Source: CAD feature listing. Evaluate the final solid. Frame: model axes, mm. Face numbers are marked on the shaded views. A direction names the side the tool comes from. Coordinates: 2 decimals unless noted, no trailing zeros. Write each loop counter-clockwise with the first axis right and the second up, starting at its lowest first coordinate (ties: lowest second). Pieces come first, ordered by that corner, then holes. Notation, with made-up numbers: (62, 61.25) -> (107, 61.25) arc R31 cw to (107, 99.25) -> close; hole circle Ø5 at (-37, 44.25). An arc over 180 degrees is marked (long way). Write item = value, one per line.
from build123d import *

# Parameters (mm, degrees)
SKIZZE1_W                       = 22.1
SKIZZE1_H                       = 4.3
SCHNITT_LINEAR_START            = -15.1
SKIZZE2_R                       = 7.5
SKIZZE2_R_2                     = 5
SCHNITT_LINEAR_AUSTRAGEN2_DEPTH = 15.1
SCHNITT_LINEAR_START_2          = -3
SCHNITT_LINEAR_AUSTRAGEN4_DEPTH = 3
AUFSATZ_LINEAR_AUSTRAGEN1_DEPTH = 1.5
DURCHGANGSLOCH_F_R_M41_D        = 4.5
VERRUNDUNG3_R                   = 2


with BuildPart() as part:
    # Skizze1 → Rotation1 (revolve)
    with BuildSketch(Plane.XY, mode=Mode.PRIVATE) as rotation1_sk:
        with Locations((11.05, 5.35)):
            Rectangle(SKIZZE1_W, SKIZZE1_H)
    revolve(rotation1_sk.sketch.rotate(Axis((0, 0, 0), (1, 0, 0)), 90), axis=Axis((0, 0, 0), (1, 0, 0)))

    # Skizze2 → Schnitt-Linear austragen2 (cut)
    with BuildSketch(Plane.ZY.offset(SCHNITT_LINEAR_START)):
        Circle(SKIZZE2_R)
        Circle(SKIZZE2_R_2, mode=Mode.SUBTRACT)
    extrude(amount=SCHNITT_LINEAR_AUSTRAGEN2_DEPTH, mode=Mode.SUBTRACT)

    # Skizze3 → Schnitt-Linear austragen4 (cut)
    with BuildSketch(Plane.ZY.offset(-15.1).offset(SCHNITT_LINEAR_START_2)):
        with BuildLine():
            Line((0, 5), (0, 7.5))
            ThreePointArc((0, 7.5), (7.451278665, -0.853490626), (-1.695892399, -7.305747667))
            Line((-1.695892399, -7.305747667), (0.652630961, -4.957224307))
            ThreePointArc((0.652630961, -4.957224307), (4.989294616, 0.327015646), (0, 5))
        make_face()
    extrude(amount=SCHNITT_LINEAR_AUSTRAGEN4_DEPTH, mode=Mode.SUBTRACT)

    # Skizze4 → Aufsatz-Linear austragen1 (add)
    with BuildSketch(Plane(origin=(22.1, 0, 0), x_dir=(0, 0, -1), z_dir=(1, 0, 0))):
        with BuildLine():
            Line((3.348469228, 6.711017347), (3.348469228, 15.5))
            Line((3.348469228, 15.5), (11.348469228, 15.5))
            Line((11.348469228, 15.5), (11.348469228, 9.5))
            Line((11.348469228, 9.5), (7.348469228, 1.5))
            ThreePointArc((7.348469228, 1.5), (5.949352783, 4.566749552), (3.348469228, 6.711017347))
        make_face()
    extrude(amount=-AUFSATZ_LINEAR_AUSTRAGEN1_DEPTH)

    # Durchgangsloch für M41 (through all)
    with Locations(Plane.ZY.offset(-18.1)):
        with Locations((-8, 11.5)):
            Hole(DURCHGANGSLOCH_F_R_M41_D / 2)

    # Verrundung3
    verrundung3_edges = [part.edges().sort_by_distance(p)[0] for p in [
        (21.35, 1.5, -7.348469228),
        (21.35, 6.711017347, -3.348469228),
        (21.35, 15.5, -3.348469228),
        (21.35, 15.5, -11.348469228),
        (21.35, 9.5, -11.348469228),
    ]]
    fillet(verrundung3_edges, radius=VERRUNDUNG3_R)


solid = part.part
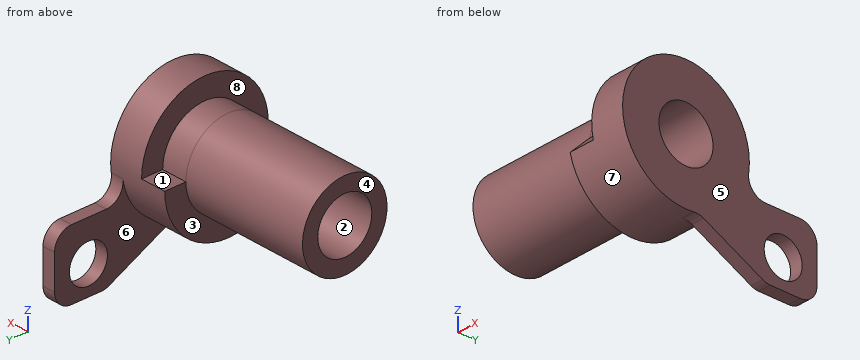
1) First-contact query: pin 1 Ø2 at (x, y) = (17.5, 6) entering from +Z; pin 2 Ø0.8 at (x, y) = (21, 12) entering from +Z; pin 3 Ø3.5 at (y, z) = (11.5, -8) entering from -X; pin 4 Ø4 at (x, z) = (11.5, 3.5) entering from +Y. Flat tips, straight axial feed; report the tip coordinate or a pass-through.
Answer block:
pin_1 = 5.4
pin_2 = -3.35
pin_3 = through
pin_4 = 4.77
2) Cut plane B-B, the plane z = -8. Output: boundary loops of the cut face in (x, y), and give its area (3 significant figures).
Answer block:
outline = (20.6, 2.8) -> (22.1, 2.8) -> (22.1, 9.25) -> (20.6, 9.25) -> close; (20.6, 13.75) -> (22.1, 13.75) -> (22.1, 15.5) -> (20.6, 15.5) -> close
area = 12.3 mm2
3) Reachability of the marked faces 4, 5, 6, 7 and 8 from +Z, -Z, +X, -X, +Y, -Y: full face, straight path, thin tool, end or side. Return the list, or none.
Answer block:
face_4 = +Z, -Z, -X, +Y, -Y
face_5 = +Z, -Z, +X, +Y, -Y
face_6 = -Z, -X, +Y
face_7 = -X
face_8 = +Z, -X
4) Cut plane C-C, the plane x = 7.25. Output: boundary loops of the cut face in (y, z).
Answer block:
outline = circle Ø10 at (0, 0); hole circle Ø6.4 at (0, 0)
5) Cut plane A-A, the plane y = 11.5. Output: boundary loops of the cut face in (x, z).
Answer block:
outline = (20.6, -11.35) -> (22.1, -11.35) -> (22.1, -10.25) -> (20.6, -10.25) -> close; (20.6, -5.75) -> (22.1, -5.75) -> (22.1, -3.35) -> (20.6, -3.35) -> close
6) Material intervals for probe 1 along Y at (x, z) = (7.75, 0); probe 2 along Z at (x, y) = (19.25, 2.75); probe 3 along Y at (x, z) = (21.15, -8), sorted ascending. Write a range as [from, to].
Answer block:
probe_1 = [-5, -3.2], [3.2, 5]
probe_2 = [-6.98, -1.64], [1.64, 6.98]
probe_3 = [2.8, 9.25], [13.75, 15.5]
7) Cut plane D-D, the plane y = 5.5. Output: boundary loops of the cut face in (x, z).
Answer block:
outline = (15.1, -5.1) -> (20.6, -5.1) -> (20.6, -9.35) -> (22.1, -9.35) -> (22.1, 5.1) -> (18.1, 5.1) -> (18.1, 0) -> (15.1, 0) -> close
8) Pull-direction query (Z, two-part tool) for the marked faces 1, 2 and 3; classes: +Z half, -Z half, draft (parallel to the pull), parting line (faces both ways), or undercut.
Answer block:
face_1 = +Z half
face_2 = undercut
face_3 = draft
